from build123d import *

# Parameters (mm, degrees)
F0_W     = 222
F0_H     = 162
F1_DEPTH = 260
F2_W     = 242
F2_H     = 182
F3_DEPTH = 2
F4_R     = 5
F5_R     = 4
F6_DEPTH = 2
F7_W     = 218
F7_H     = 158
F8_DEPTH = 258


with BuildPart() as f1:
    # F0 (on Top) → F1 (new body)
    with BuildSketch(Plane.XY):
        Rectangle(F0_W, F0_H)
    extrude(amount=F1_DEPTH)

    # F2 (on face) → F3 (join)
    with BuildSketch(Plane(origin=(0, 0, 0), x_dir=(1, 0, 0), z_dir=(0, 0, -1))):
        Rectangle(F2_W, F2_H)
    extrude(amount=F3_DEPTH)

    # F4
    f4_edges = [f1.edges().sort_by_distance(p)[0] for p in [
        (0, -81, 260),
        (111, 0, 260),
        (0, 81, 260),
        (-111, 0, 260),
        (111, -81, 130),
        (-111, -81, 130),
        (111, 81, 130),
        (-111, 81, 130),
    ]]
    fillet(f4_edges, radius=F4_R)

    # F7 (on face) → F8 (cut)
    with BuildSketch(Plane(origin=(0, 0, -2), x_dir=(1, 0, 0), z_dir=(0, 0, -1))):
        Rectangle(F7_W, F7_H)
    extrude(amount=-F8_DEPTH, mode=Mode.SUBTRACT)


with BuildPart() as f6:
    # F5 (on Right) → F6 (new body)
    with BuildSketch(Plane.YZ):
        with BuildLine():
            Line((-101, 20.151517), (-81, 20.151517))
            Line((-81, 20.151517), (-81, 40.151517))
            Line((-81, 40.151517), (-101, 40.151517))
            ThreePointArc((-101, 40.151517), (-111, 30.151517), (-101, 20.151517))
        make_face()
        with Locations((-101, 30.151517)):
            Circle(F5_R, mode=Mode.SUBTRACT)
    extrude(amount=F6_DEPTH)


solid = f1.part
Input: part model. Units: mm. Frame: model coordinates. A direction names the side the tool comes from. Round coordinates to 2 decimals unless told otherwise and drop trailing zeros. Write each loop counter-clockwise with the first axis right and the second up, starting at its lowest first coordinate (ties: lowest second). Pieces come first, ordered by that corner, then holes.
1) Cut plane C-C (x = 95). Return the cut outline in (y, z), then the cut area to 3 significant figures.
2) Draft query along Y for faces 6 (the flat face through (-1, 1, 260)), 7 (the flat face through (-2, 79, 125)), 8 (the flat face through (-1, -81, 126)). Return one class per face: pulls with the +Y half, pulls with the -Y half, needs draft (parallel to the pull), parting line crosses it, or undercut.
3) Reachability of faces 1 (the flat face through (-0.6, -81.3, 0)), 2 (the flat face through (-111, -1, 126)), 3 (the flat face through (-109, 1, 125)), 4 (the flat face through (-1, 81, 126)), 5 (the flat face through (111, -1, 126)) from +Z, -Z, +X, -X, +Y, -Y: full face, straight path, thin tool, end or side. Return the list, or none.
4) Cut plane A-A (z = 15.5). Return the cut outline in (x, y), then the cut area to 3 significant figures.
5) Contact query for flat-ended pins moving along their axis: P1, Ø6, axis at x = -61, z = 221.5, coming from the -Y side; P2, Ø1, axis at x = -60, z = 162, coming from the +Y side; P3, Ø8, axis at x = 5, y = 43.5, coming from the -Z side. Output: stop coordinate, or through.
6) Ray query, L1, parallel to X at y = 44.5, z = 116; L2, parallel to Y at x = -97.5, z = 163; L3, parallel to Y at x = -110, z = 54.5. Return the intervals inside material, ascending.
7) Cut plane B-B (y = -66). Return the cut outline in (x, z), then the cut area to 3 significant figures.
Geometry says:
1. outline: (-91, -2) - (-79, -2) - (-79, 256) - (79, 256) - (79, -2) - (91, -2) - (91, 0) - (81, 0) - (81, 255) arc R5 ccw to (76, 260) - (-76, 260) arc R5 ccw to (-81, 255) - (-81, 0) - (-91, 0) - close
1. area: 1,710 mm2
2. face 6: needs draft
2. face 7: undercut
2. face 8: pulls with the -Y half
3. face 1: +Z
3. face 2: +Z, -X, +Y, -Y
3. face 3: -Z
3. face 4: +Z, +X, -X, +Y
3. face 5: +Z, +X, +Y, -Y
4. outline: (-111, -76) arc R5 ccw to (-106, -81) - (106, -81) arc R5 ccw to (111, -76) - (111, 76) arc R5 ccw to (106, 81) - (-106, 81) arc R5 ccw to (-111, 76) - close; hole (-109, -79) - (109, -79) - (109, 79) - (-109, 79) - close
4. area: 1,500 mm2
5. P1: stops at y = -81
5. P2: stops at y = 81
5. P3: stops at z = 256
6. L1: x = -111 to -109, 109 to 111
6. L2: y = -81 to -79, 79 to 81
6. L3: y = -79 to 79
7. outline: (-121, -2) - (-109, -2) - (-109, 256) - (109, 256) - (109, -2) - (121, -2) - (121, 0) - (111, 0) - (111, 255) arc R5 ccw to (106, 260) - (-106, 260) arc R5 ccw to (-111, 255) - (-111, 0) - (-121, 0) - close
7. area: 1,950 mm2
